Read the model definition and answer for the solid it produces. Units are mm, in the model's axes. Give positions to 0.01 mm unless a question says otherwise; leave off trailing zeros. Order: outer loops, then holes, each group sorted by start corner. A loop starts at its lowest first (then second) coordinate and runs counter-clockwise, first axis right, second up. Notation, with made-up numbers: (79.25, -21) - (86.25, -21) arc R28 ccw to (86.25, 8) - close; hole circle Ø2 at (28.25, 9). An arc over 180 degrees is marked (long way). Write each question's results on one line, items separated by ' | '. Start each with the question number.
Q1. Find section B-B on x = 35. Give the vertices of the cut face in (y, z).
Q2. Flat-ended cylindrical pins translate along their axes: P1, Ø4, axis at x = 60.5, y = 3, coming from the -Z side; P2, Ø2.5, axis at x = 35, z = -68, coming from the -Y side. Find the tip coordinate at first contact, or state that the pin passes through.
Q3. Find the intervals of material crossed by line 1 along Z through (x, y) = (35, 2.5); line 2 along X through (y, z) = (4.25, -61); line 3 along X through (y, z) = (7.75, -59.5), in increasing order. Write a range as from..to.
Q4. Find section A-A on z = -68. Give the vertices of the cut face in (x, y).
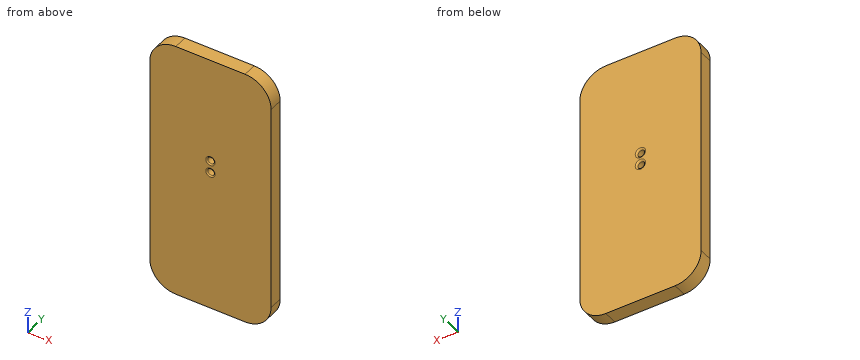
Autodesk Inventor part; units mm, degrees
ref_plane "YZ Plane" through (0, 0, 0) normal (1, 0, 0) x (0, 1, 0)
ref_plane "XZ Plane" through (0, 0, 0) normal (0, 1, 0) x (-1, 0, 0)
ref_plane "XY Plane" through (0, 0, 0) normal (0, 0, 1) x (1, 0, 0)
sketch "Esboço4" plane through (0, 0, 0) normal (0, 1, 0) x (-1, 0, 0)
  line L0 (0, -15) -> (0, -135)
  line L1 (-15, -150) -> (-55, -150)
  line L2 (-70, -135) -> (-70, -15)
  line L3 (-55, 0) -> (-15, 0)
  arc A0 (-15, -150) -> (0, -135) centre (-15, -135) ccw
  arc A1 (-70, -135) -> (-55, -150) centre (-55, -135) ccw
  arc A2 (-55, 0) -> (-70, -15) centre (-55, -15) ccw
  arc A3 (0, -15) -> (-15, 0) centre (-15, -15) ccw
  point P0 (0, 0)
  point P1 (0, -150)
  point P2 (-70, -150)
  dimension "d7" = 150
  dimension "d8" = 70
  dimension "d9" = 15
extrude "Extrusão2" add sketch "Esboço4" along normal blind 8
sketch "Esboço5" plane through (0, 8, 0) normal (0, 1, 0) x (1, 0, 0)
  line L0 (15, 0) -> (55, 0)
  line L1 (55, 150) -> (15, 150)
  circle A0 centre (35, 68) radius 2
  circle A1 centre (35, 61) radius 2
  point P0 (0, 0)
  dimension "d13" = 4
  dimension "d15" = 4
extrude "Extrusão3" cut sketch "Esboço5" against normal through all
fillet "Arredondamento1" radius 1 2 edges at (33, 8, -68) (33, 8, -61)
fillet "Arredondamento2" radius 0.7 2 edges at (33, 0, -61) (33, 0, -68)
properties part number "Base superior(suporte)" material "ABS plástico"
Working result:
1) outline: (0, -150) - (8, -150) - (8, -71) arc R1 ccw to (7, -70) - (0.7, -70) arc R0.7 ccw to (0, -70.7) - close; (0, -65.3) arc R0.7 ccw to (0.7, -66) - (7, -66) arc R1 ccw to (8, -65) - (8, -64) arc R1 ccw to (7, -63) - (0.7, -63) arc R0.7 ccw to (0, -63.7) - close; (0, -58.3) arc R0.7 ccw to (0.7, -59) - (7, -59) arc R1 ccw to (8, -58) - (8, 0) - (0, 0) - close
2) P1: z = -149.59 | P2: through
3) line 1: -150..-70, -66..-63, -59..0 | line 2: 0..33, 37..70 | line 3: 0..33.21, 36.79..70
4) outline: (0, 0) - (32.3, 0) arc R0.7 ccw to (33, 0.7) - (33, 7) arc R1 ccw to (32, 8) - (0, 8) - close; (37, 0.7) arc R0.7 ccw to (37.7, 0) - (70, 0) - (70, 8) - (38, 8) arc R1 ccw to (37, 7) - close
